Autodesk Inventor part; units mm, degrees
ref_plane "YZ Plane" through (0, 0, 0) normal (1, 0, 0) x (0, 1, 0)
ref_plane "XZ Plane" through (0, 0, 0) normal (0, 1, 0) x (-1, 0, 0)
ref_plane "XY Plane" through (0, 0, 0) normal (0, 0, 1) x (1, 0, 0)
ref_plane "Work Plane1" through (0, 0, 0) normal (0, 0, 1) x (1, 0, 0)
sketch "Sketch1" plane through (0, 0, 0) normal (0, 0, 1) x (1, 0, 0)
  arc A0 (-12, 16) -> (-12, 24) centre (-12, 20) ccw
  line L0 (-12, 3) -> (-12, 16)
  line L1 (0, 3) -> (-12, 3)
  line L2 (0, 3) -> (0, 30)
  line L3 (-12, 30) -> (0, 30)
  line L4 (-12, 24) -> (-12, 30)
  circle A1 centre (-12, 20) radius 4
  circle A2 centre (-12, 20) radius 17.5
  line L5 (-12, 20) -> (0, 20)
  line L6 (0, 20) -> (0, 320)
  line L7 (0, 320) -> (-12, 320)
  line L8 (-12, 320) -> (-12, 20)
  line L9 (-12, 320) -> (-24, 320)
  line L10 (-24, 320) -> (-24, 20)
  line L11 (-24, 20) -> (-12, 20)
  line L12 (-12, 20) -> (-12, 320)
  point P0 (0, 0)
  point P1 (0, 32.7377)
  point P2 (-24, 32.7377)
  dimension "d0" = 35
  dimension "d1" = 300
  dimension "d2" = 12
extrude "Extrusion1" add sketch "Sketch1" along normal blind 12 contours A0 L5 L2 A2 L1 L0 | L0 L1 A2 L10 L11 A1 | A0 L4 L3 L2 L5 | L11 L10 A2 L8 L4 A1 | L2 L6 A2 | L8 A2 L6 L3 | L10 L9 L8 A2 | L8 L7 L6 A2
fillet "Fillet1" radius 10 2 edges at (-24, 32.7377, 6) (0, 32.7377, 6)
mirror "Mirror1" about plane through (0, 320, 0) normal (0, 1, 0) of "Extrusion1"
properties part number "arm"
Here's how the part is built. I have some questions about the finished solid (model axes, mm). A direction names the side the tool comes from. Give positions to 0.01 mm unless a question says otherwise; leave off trailing zeros. Order: outer loops, then holes, each group sorted by start corner. A loop starts at its lowest first (then second) coordinate and runs counter-clockwise, first axis right, second up. Notation, with made-up numbers: (-29, 2) -> (-19, 2) arc R25 cw to (-19, 21) -> close; hole circle Ø11 at (76, 38). An arc over 180 degrees is marked (long way). Use CSV: the item, a comma, the result in double quotes. Start each with the question number.
Item 1: If I drill on probe 1 along Y at (x, z) = (-12, 5.5); probe 2 along Y at (x, z) = (-14.5, 4.75); probe 3 along X at (y, z) = (20, 4.25), over which ranges is the centre line in solid material (lowest first)? Write a range as [from, to].
Item 2: Suppose I cut it at B-B (y = 115.5). List the corners of the cut face in (x, z) for me.
Item 3: Suppose I cut it at A-A (z = 5). List the corners of the cut face in (x, y) for me, and give its area (3 significant figures).
Item 4: On a 3-axis mill with a long thin cutter (end or side, diameter ignored), from which of +Z, -Z, +X, -X, +Y, -Y can I reach the whole of each face in a straight line? I mean faces 3 (the flat face through (0, 318, 6)), 4 (the flat face through (-24, 326, 6)), 5 (the flat face through (-12, 324, 12)). Say none if no direction works.
Item 5: Thinking about a two-plate mould opening in Y: for faces 1 (the flat face through (-12, 324, 0)), 2 (the cylindrical face through (-12.58, 637.49, 5.92)), which applies, pulls with the +Y half, pulls with the -Y half, needs draft (parallel to the pull), parting line crosses it, or undercut?
Item 6: I'm going to push flat-ended pins straight in: P1, Ø1.5, axis at y = 147.5, z = 10, coming from the -X side; P2, Ø3, axis at x = -18, z = 4, coming from the +Y side; P3, Ø3, axis at x = -14, z = 4, coming from the +Y side; P4, Ø7, axis at x = -12, y = 20, coming from the +Z side. Where does each tip first touch, or does it pass through?
Answer block:
1,probe 1,"y = [2.5, 16], [24, 616], [624, 637.5]"
1,probe 2,"y = [2.68, 16.88], [23.12, 616.88], [623.12, 637.32]"
1,probe 3,"x = [-29.5, -16], [-8, 5.5]"
2,outline,"(-24, 0) -> (0, 0) -> (0, 12) -> (-24, 12) -> close"
3,outline,"(-26, 30.5) arc R17.5 ccw (long way) to (2, 30.5) arc R10 cw to (0, 36.5) -> (0, 607.26) arc R17.5 ccw (long way) to (-24, 607.26) -> (-24, 36.5) arc R10 cw to start; hole circle Ø8 at (-12, 20); hole circle Ø8 at (-12, 620)"
3,area,"15,500 mm^2"
4,face 3,"+Z, -Z, +X"
4,face 4,"+Z, -Z, -X"
4,face 5,"+Z, +X, -X, +Y, -Y"
5,face 1,"needs draft"
5,face 2,"undercut"
6,P1,"stops at x = -24"
6,P2,"stops at y = 636.91"
6,P3,"stops at y = 637.49"
6,P4,"passes through"
